The model under review builds one solid part; all positions refer to its coordinate system, in mm. Round coordinates to 2 decimals unless told otherwise and drop trailing zeros. Loops run counter-clockwise (first coordinate to the right, second up) from the corner with the lowest first, then second, coordinate; pieces in that order, holes last. Notation, with made-up numbers: M -38.5,48.5 L -16.5,48.5 A28 ccw -16.5,66.5 Z; hole C 85,31.5 d1. An arc over 180 degrees is marked long. Answer as a JSON object with one key per item and string values. Group by question number.
Item 1: Consider section B-B (x = 552.5). Give the boundary of the cut face in (y, z), and give its area (3 significant figures).
Item 2: Consider section A-A (y = 757.5). Give the boundary of the cut face in (x, z) (3 decimals), and give its area (3 significant figures).
Item 3: The part is to be moulded in two halves that separate along X. For faces 1 (the face through (-3.175, 398, 18)), 2 (the face through (787, 398, -3.175)), 3 (the face through (398, 398, 0)), say which applies: +X half, -X half, draft (parallel to the pull), parting line (faces both ways), or undercut.
Item 4: Insertion check: P1, Ø5, axis at y = 341.5, z = 42.5, coming from the +X side; P2, Ø8, axis at x = 141, z = 3, coming from the -Y side; P3, Ø1.6, axis at x = -1.5, y = 411.5, coming from the +Z side; P4, Ø1.9, axis at y = 370, z = 40.5, coming from the -X side. Each pin has a flat end and moves straight along its axis. Give the tip position at first contact, or say it passes through.
Item 5: To check wall thickness, follow line 1 (Z direction, x = 216, y = 330); line 2 (X direction, y = 214, z = 40). State the ranges of each line that lie inside material, in increasing order.
```python
from build123d import *

# Parameters (mm, degrees)
F0_W     = 806.45
F0_H     = 44.45
F1_DEPTH = 806.45
F3_DEPTH = 806.45


with BuildPart() as f1:
    # F0 (on Front) → F1 (new body)
    with BuildSketch(Plane.XZ):
        with Locations((403.225, 22.225)):
            Rectangle(F0_W, F0_H)
    extrude(amount=-F1_DEPTH)

    # F2 (on Front) → F3 (join)
    with BuildSketch(Plane.XZ):
        Polygon((-3.175, -3.175), (0, -3.175), (41.275, -3.175), (41.275, 0), (0, 0), (0, 38.1), (-3.175, 38.1), align=None)
        Polygon((765.175, -3.175), (806.45, -3.175), (809.625, -3.175), (809.625, 38.1), (806.45, 38.1), (806.45, 0), (765.175, 0), align=None)
    extrude(amount=-F3_DEPTH)


solid = f1.part
```
Geometry results:
{
 "1": {"outline": "M 0,0 L 806.45,0 L 806.45,44.45 L 0,44.45 Z", "area": "35,800 mm^2"},
 "2": {"outline": "M -3.175,-3.175 L 41.275,-3.175 L 41.275,0 L 765.175,0 L 765.175,-3.175 L 809.625,-3.175 L 809.625,38.1 L 806.45,38.1 L 806.45,44.45 L 0,44.45 L 0,38.1 L -3.175,38.1 Z", "area": "36,400 mm^2"},
 "3": {"face 1": "-X half", "face 2": "draft", "face 3": "undercut"},
 "4": {"P1": "stops at x = 806.45", "P2": "stops at y = 0", "P3": "stops at z = 38.1", "P4": "stops at x = 0"},
 "5": {"line 1": "z = 0 to 44.45", "line 2": "x = 0 to 806.45"}
}
